from build123d import *

# Parameters (mm, degrees)
SZKIC1_W                    = 51
SZKIC1_H                    = 60
SZKIC1_R                    = 4.5
SZKIC1_R_2                  = 10
DODANIE_WYCI_GNI_CIE1_DEPTH = 5
DODANIE_WYCI_GNI_CIE2_START = 5
SZKIC2_W                    = 51
SZKIC2_H                    = 48
SZKIC2_R                    = 13
DODANIE_WYCI_GNI_CIE2_DEPTH = 10
ZAOKR_GLENIE1_R             = 25


with BuildPart() as part:
    # Szkic1 → Dodanie-wyciągnięcie1 (new body)
    with BuildSketch(Plane(origin=(0, 0, 0), x_dir=(1, 0, 0), z_dir=(0, 1, 0))):
        Rectangle(SZKIC1_W, SZKIC1_H)
        with Locations(Location((0, 24, 0), (0, 0, 270))):
            Circle(SZKIC1_R, mode=Mode.SUBTRACT)
        with Locations(Location((0, -15, 0), (0, 0, 270))):
            Circle(SZKIC1_R_2, mode=Mode.SUBTRACT)
    extrude(amount=DODANIE_WYCI_GNI_CIE1_DEPTH)

    # Szkic2 → Dodanie-wyciągnięcie2 (add)
    with BuildSketch(Plane(origin=(0, 0, 0), x_dir=(1, 0, 0), z_dir=(0, 1, 0)).offset(DODANIE_WYCI_GNI_CIE2_START)):
        with Locations((0, -6)):
            Rectangle(SZKIC2_W, SZKIC2_H)
        with Locations(Location((0, -15, 0), (0, 0, 270))):
            Circle(SZKIC2_R, mode=Mode.SUBTRACT)
    extrude(amount=DODANIE_WYCI_GNI_CIE2_DEPTH)

    # Zaokrąglenie1
    zaokr_glenie1_edges = [part.edges().sort_by_distance(p)[0] for p in [
        (25.5, 7.5, 30),
        (-25.5, 7.5, 30),
    ]]
    fillet(zaokr_glenie1_edges, radius=ZAOKR_GLENIE1_R)


solid = part.part
The listing builds one solid part. Answer for the finished solid, in the listing's coordinates (mm). A direction names the side the tool comes from. Round coordinates to 2 decimals unless told otherwise and drop trailing zeros. Write each loop counter-clockwise with the first axis right and the second up, starting at its lowest first coordinate (ties: lowest second). Pieces come first, ordered by that corner, then holes. Notation, with made-up numbers: (-7.5, -36) - (31.5, -36) arc R12 cw to (31.5, -14) - close; hole circle Ø9 at (33.5, -27.75). An arc over 180 degrees is marked (long way). Use one line per item in the form item = value. Start each with the question number.
Item 1: Flat-ended cylindrical pins translate along their axes: pin 1 Ø3 at (x, y) = (10, 6) entering from +Z; pin 2 Ø1 at (y, z) = (8, 15) entering from +X; pin 3 Ø13 at (x, z) = (-1.5, 19) entering from +Y; pin 4 Ø1 at (x, z) = (7.5, 13) entering from -Y. Find the tip coordinate at first contact, or state that the pin passes through.
Item 2: A cutting plane is placed at A-A (z = -24). Write down the section's boundary in (x, y).
Item 3: A cutting plane is placed at D-D (x = -8). Write down the section's boundary in (y, z), plus the area to 3 significant figures.
Item 4: A cutting plane is placed at C-C (y = 4). Write down the section's boundary in (x, z), plus the area to 3 significant figures.
Item 5: Determine the mould class of faces 1 (the flat face through (-25.5, 7, -8)), 2 (the cylindrical face through (0.198, 2.465, -28.496)), 3 (the flat face through (0, 10, -18)) for opening direction Z: +Z half, -Z half, draft (parallel to the pull), parting line (faces both ways), or undercut.
Item 6: Find the intervals of material crossed by line 1 (X direction, y = 12.5, z = 15); line 2 (X direction, y = 1.85, z = 15); line 3 (Y direction, x = -20, z = -22), in increasing order. Write a range as [from, to].
Item 7: A tool of negligible diameter and unlimited length cuts with its end or side. For faces 4 (the flat face through (0, 5, -19)), 5 (the flat face through (0, 0, 0)), 6 (the flat face through (7, 5, 23)), from which of +Z, -Z, +X, -X, +Y, -Y can it reach the whole face along a straight path? Write none if from no direction.
Item 8: A cutting plane is placed at B-B (y = 13.75). Write down the section's boundary in (x, z).
The answers:
q1.pin_1 = 28.69
q1.pin_2 = 23.62
q1.pin_3 = 5
q1.pin_4 = through
q2.outline = (-25.5, 0) - (-4.5, 0) - (-4.5, 5) - (-25.5, 5) - close; (4.5, 0) - (25.5, 0) - (25.5, 5) - (4.5, 5) - close
q3.outline = (0, -30) - (5, -30) - (5, -18) - (15, -18) - (15, 4.75) - (5, 4.75) - (5, 9) - (0, 9) - close; (0, 21) - (5, 21) - (5, 25.25) - (15, 25.25) - (15, 28.85) - (0, 28.85) - close
q3.area = 498 mm^2
q4.outline = (-25.5, -30) - (25.5, -30) - (25.5, 5) arc R25 ccw to (0.5, 30) - (-0.5, 30) arc R25 ccw to (-25.5, 5) - close; hole circle Ø20 at (0, 15); hole circle Ø9 at (0, -24)
q4.area = 2,410 mm^2
q5.face_1 = draft
q5.face_2 = undercut
q5.face_3 = -Z half
q6.line_1 = [-23.41, -13], [13, 23.41]
q6.line_2 = [-23.41, -10], [10, 23.41]
q6.line_3 = [0, 5]
q7.face_4 = -Z, +X, -X, +Y
q7.face_5 = +Z, -Z, +X, -X, -Y
q7.face_6 = +Y
q8.outline = (-25.5, -18) - (25.5, -18) - (25.5, 5) arc R25 ccw to (0.5, 30) - (-0.5, 30) arc R25 ccw to (-25.5, 5) - close; hole circle Ø26 at (0, 15)
